Design review of the part shown in the three views and the two pictorial views. Dimensions are in mm from the part's minimum x, y and z. A direction names the side the tool comes from. Round coordinates to 2 decimals unless told otherwise and drop trailing zeros. Loops run counter-clockwise (first coordinate to the right, second up) from the corner with the lowest first, then second, coordinate; pieces in that order, holes last. Notation, with made-up numbers: M -10,-39.75 L 7,-39.75 A11 ccw 7,-29.75 Z; hole C 18.25,-24.5 d6. An arc over 180 degrees is marked long. One line per question, with ' | ' between items.
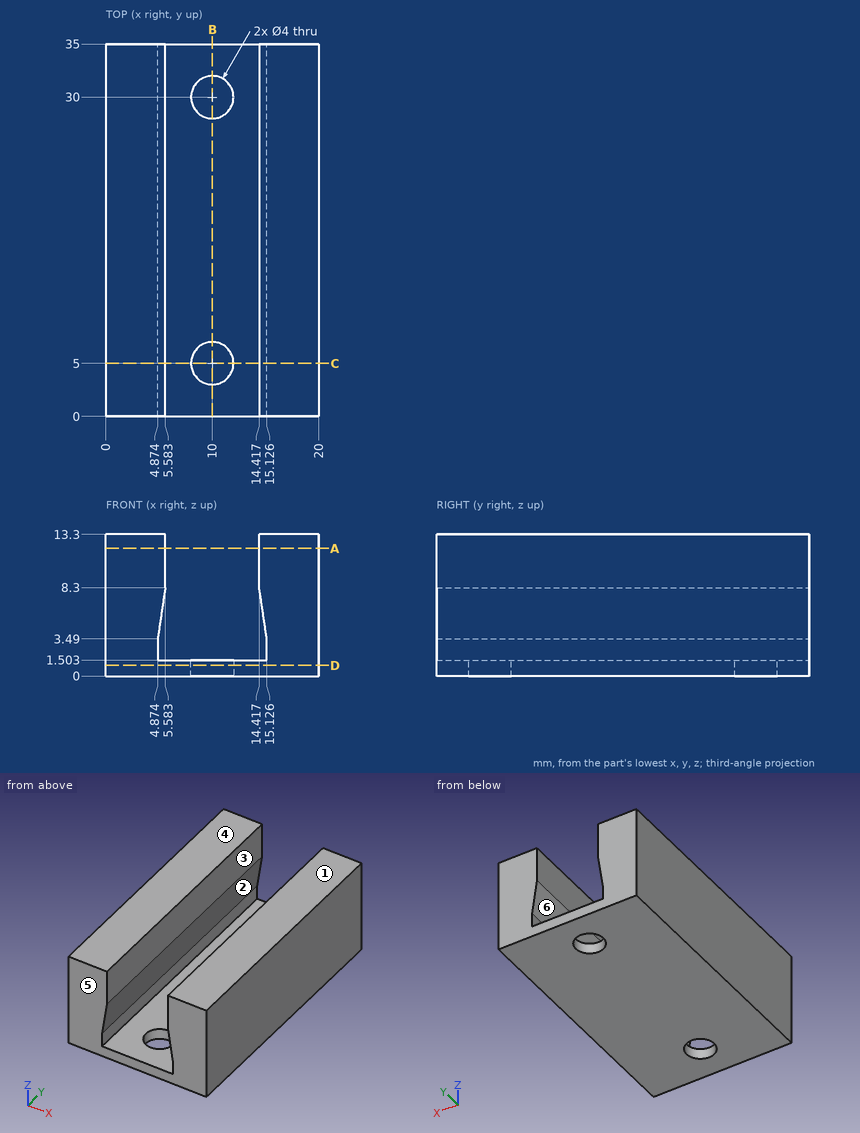
1) Add section B-B on x = 10. State the section outline as (y, z) points.
Output values:
outline: M 0,0 L 3,0 L 3,1.5 L 0,1.5 Z; M 7,0 L 28,0 L 28,1.5 L 7,1.5 Z; M 32,0 L 35,0 L 35,1.5 L 32,1.5 Z
2) For line 1 (Y direction, x = 10, z = 0.95); line 2 (X direction, y = 16.5, z = 10); line 3 (X direction, y = 32.5, z = 3.5) (1 decimal), list the stretches that pass through material, from the lowest coordinate up.
Output values:
line 1: y = 0 to 3, 7 to 28, 32 to 35 | line 2: x = 0 to 5.58, 14.42 to 20 | line 3: x = 0 to 4.9, 15.1 to 20
3) Mouldability with a two-part tool opening along Z and no side actions: class the marked faces 4, 5 and 6 as +Z half, -Z half, draft (parallel to the pull), parting line (faces both ways), or undercut.
Output values:
face 4: +Z half | face 5: draft | face 6: undercut
4) Machinability: for the marked faces 1, 2 and 3, which of the approach directions +Z, -Z, +X, -X, +Y, -Y give a long, thin tool a straight path to every point of the face, cutting with its end or side? Answer none if there is none.
Output values:
face 1: +Z, +X, -X, +Y, -Y | face 2: +Y, -Y | face 3: +Z, +Y, -Y
5) Add section D-D on z = 1. State the section outline as (x, y) points.
Output values:
outline: M 0,0 L 20,0 L 20,35 L 0,35 Z; hole C 10,5 d4; hole C 10,30 d4
6) Add section C-C on y = 5. State the section outline as (x, z) points.
Output values:
outline: M 0,0 L 8,0 L 8,1.5 L 4.87,1.5 L 4.87,3.49 L 5.58,8.3 L 5.58,13.3 L 0,13.3 Z; M 12,0 L 20,0 L 20,13.3 L 14.42,13.3 L 14.42,8.3 L 15.13,3.49 L 15.13,1.5 L 12,1.5 Z
7) Add section A-A on z = 12. State the section outline as (x, y) points, then the cut area to 3 significant figures.
Output values:
outline: M 0,0 L 5.58,0 L 5.58,35 L 0,35 Z; M 14.42,0 L 20,0 L 20,35 L 14.42,35 Z | area: 391 mm²
8) Insertion check: P1, Ø2.5, axis at x = 10, y = 30, coming from the -Z side; P2, Ø2, axis at x = 17.5, y = 18, coming from the -Z side; P3, Ø3, axis at x = 8, y = 10, coming from the +Z side. Each pin has a flat end and moves straight along its axis. Give the tip position at first contact, or say it passes through.
Output values:
P1: passes through | P2: stops at z = 0 | P3: stops at z = 1.5
